The listing builds one solid part. Answer for the finished solid, in the listing's coordinates (mm). Face numbers are marked on the shaded views. A direction names the side the tool comes from. Coordinates: 2 decimals unless noted, no trailing zeros. Write each loop counter-clockwise with the first axis right and the second up, starting at its lowest first coordinate (ties: lowest second). Pieces come first, ordered by that corner, then holes. Notation, with made-up numbers: M 9.5,87.5 L 40.5,87.5 A22 cw 40.5,104.5 Z; hole C 15.5,83.25 d1. An arc over 180 degrees is marked long. Put each result on its own line as item: value. Start each with the question number.
```python
from build123d import *

# Parameters (mm, degrees)
BOSS_EXTRUDE1_DEPTH      = 1400
BOSS_EXTRUDE1_DEPTH_BACK = 400
SKETCH1_R                = 125
BOSS_EXTRUDE2_DEPTH      = 50


with BuildPart() as part:
    # Sketch1 → Boss-Extrude1 (new, two sides: drawn at the far end of the back side and taken through both)
    with BuildSketch(Plane(origin=(0, 0, 0), x_dir=(1, 0, 0), z_dir=(0, 1, 0)).offset(-BOSS_EXTRUDE1_DEPTH_BACK)):
        with Locations(Location((0, 0, 0), (0, 0, 270))):
            Circle(SKETCH1_R)
    extrude(amount=BOSS_EXTRUDE1_DEPTH + BOSS_EXTRUDE1_DEPTH_BACK)

    # Sketch2 → Boss-Extrude2 (add, symmetric)
    with BuildSketch(Plane.XY):
        with BuildLine():
            ThreePointArc((49.472820857, 1522.279340233), (0, 1479.520886781), (-49.472820857, 1522.279340233))
            Line((-49.472820857, 1522.279340233), (-125, 1400))
            Line((-125, 1400), (125, 1400))
            Line((125, 1400), (49.472820857, 1522.279340233))
        make_face()
        with BuildLine():
            ThreePointArc((45, 1529.520886781), (0, 1484.520886781), (-45, 1529.520886781))
            Line((-45, 1529.520886781), (-49.472820857, 1522.279340233))
            ThreePointArc((-49.472820857, 1522.279340233), (0, 1479.520886781), (49.472820857, 1522.279340233))
            Line((49.472820857, 1522.279340233), (45, 1529.520886781))
        make_face()
        with BuildLine():
            Line((-49.472820857, 1522.279340233), (-45, 1529.520886781))
            ThreePointArc((-45, 1529.520886781), (0, 1574.520886781), (45, 1529.520886781))
            Line((45, 1529.520886781), (49.472820857, 1522.279340233))
            ThreePointArc((49.472820857, 1522.279340233), (49.868031056, 1525.890531625), (50, 1529.520886781))
            ThreePointArc((50, 1529.520886781), (-3.630355157, 1579.388917838), (-49.472820857, 1522.279340233))
        make_face()
    extrude(amount=BOSS_EXTRUDE2_DEPTH, both=True)


solid = part.part
```
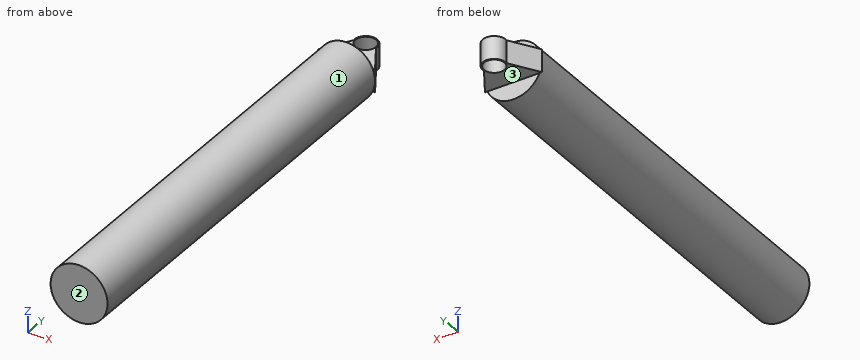
1) A cutting plane is placed at A-A on x = 0. Write down the section's boundary in (y, z), then the cut area to 3 significant figures.
2) A cutting plane is placed at B-B on z = 23. Write down the section's boundary in (x, y), then the cut area to 3 significant figures.
3) A cutting plane is placed at C-C on y = 1426.5. Write down the section's boundary in (x, z).
4) For the marked faces 1, 2 and 3, determine the directions among +Z, -Z, +X, -X, +Y, -Y from which every point of the face is accessible in a straight line to the end or side of a thin tool.
5) Given pin 1 Ø10 at (y, z) = (105.5, 24.5) entering from -X; pin 2 Ø1.5 at (x, z) = (33, 87.5) entering from +Y; pin 3 Ø6 at (x, y) = (24.5, 820.5) entering from +Z, each flat-ended and moving along its own axis, determine where each tip first touches the part or whether it passes through.
6) Straight lines are drawn through the part: probe 1 along Y at (x, z) = (0, 3); probe 2 along Y at (x, z) = (5, 45); probe 3 along Y at (x, z) = (-20, 53.5). For each, find the intervals that lie inside material, in ascending order.
7) A cutting plane is placed at D-D on z = -86.5. Write down the section's boundary in (x, y), then the cut area to 3 significant figures.
Answers follow:
1. outline: M -400,-125 L 1400,-125 L 1400,-50 L 1484.52,-50 L 1484.52,50 L 1400,50 L 1400,125 L -400,125 Z; M 1574.52,-50 L 1579.52,-50 L 1579.52,50 L 1574.52,50 Z
1. area: 459,000 mm²
2. outline: M -125,1400 L -122.87,1400 L -122.87,-400 L 122.87,-400 L 122.87,1400 L 125,1400 L 49.47,1522.28 A50 ccw long -49.47,1522.28 Z; hole C 0,1529.52 d90
2. area: 462,000 mm²
3. outline: M -108.63,-50 L 108.63,-50 L 108.63,50 L -108.63,50 Z
4. face 1: -Y
4. face 2: +Z, -Z, +X, -X, -Y
4. face 3: -Z, +X, -X, +Y
5. pin 1: stops at x = -123.47
5. pin 2: stops at y = 1400
5. pin 3: stops at z = 123.14
6. probe 1: y = -400 to 1484.52, 1574.52 to 1579.52
6. probe 2: y = -400 to 1484.8, 1574.24 to 1579.27
6. probe 3: y = -400 to 1400
7. outline: M -90.24,-400 L 90.24,-400 L 90.24,1400 L -90.24,1400 Z
7. area: 325,000 mm²
